Here's how the part is built. I have some questions about the finished solid (model axes, mm). Coordinates: 2 decimals unless noted, no trailing zeros. Write each loop counter-clockwise with the first axis right and the second up, starting at its lowest first coordinate (ties: lowest second). Pieces come first, ordered by that corner, then holes.
```python
from build123d import *

# Parameters (mm, degrees)
BOSS_EXTRUDE1_DEPTH      = 195
BOSS_EXTRUDE1_DEPTH_BACK = 195
BOSS_EXTRUDE1_START      = -20000
SKETCH1_W                = 640
SKETCH1_H                = 390
SKETCH2_W                = 300
SKETCH2_H                = 350
CUT_EXTRUDE1_DEPTH       = 20207.079530676
SKETCH3_W                = 290
SKETCH3_H                = 20
SKETCH3_W_2              = 600
SKETCH3_H_2              = 190
CUT_EXTRUDE2_DEPTH       = 20202.300081925
FILLET1_R                = 50
FILLET2_R                = 10
FILLET4_R                = 100


# Some blends are built 0.0001 mm under size
with BuildPart() as part:
    # Sketch1 → Boss-Extrude1 (new, two sides: drawn at the far end of the back side and taken through both)
    with BuildSketch(Plane.XY.offset(BOSS_EXTRUDE1_START - BOSS_EXTRUDE1_DEPTH_BACK)):
        Rectangle(SKETCH1_W, SKETCH1_H)
    extrude(amount=BOSS_EXTRUDE1_DEPTH + BOSS_EXTRUDE1_DEPTH_BACK)

    # Sketch2 → Cut-Extrude1 (cut, through all)
    with BuildSketch(Plane(origin=(320, 0, 0), x_dir=(0, 0, -1), z_dir=(1, 0, 0))):
        with Locations((20095, 0)):
            Rectangle(SKETCH2_W, SKETCH2_H)
    extrude(amount=-CUT_EXTRUDE1_DEPTH, mode=Mode.SUBTRACT)

    # Sketch3 → Cut-Extrude2 (cut, through all)
    with BuildSketch(Plane.XZ.offset(195)):
        with Locations((-155, -20165)):
            Rectangle(SKETCH3_W, SKETCH3_H)
        with Locations((155, -20165)):
            Rectangle(SKETCH3_W, SKETCH3_H)
        with Locations((0, -20040)):
            Rectangle(SKETCH3_W_2, SKETCH3_H_2)
    extrude(amount=-CUT_EXTRUDE2_DEPTH, mode=Mode.SUBTRACT)

    # Fillet1
    # the kernel refuses this fillet: 50 mm, written as the material it adds along each edge
    with BuildSketch(Plane(origin=(300, -195, -20135), x_dir=(-1, 0, 0), z_dir=(0, 1, 0)), Plane(origin=(-300, -195, -20135), x_dir=(0, 0, 1), z_dir=(0, 1, 0)), Plane(origin=(300, 175, -19945), x_dir=(0, 0, -1), z_dir=(0, 1, 0)), Plane(origin=(-300, -175, -19945), x_dir=(0, 1, 0), z_dir=(-1, 0, 0)), Plane(origin=(320, -175, -19945), x_dir=(0, 1, 0), z_dir=(-1, 0, 0)), Plane(origin=(-300, -195, -19945), x_dir=(1, 0, 0), z_dir=(0, 1, 0))) as fillet1_piece_1:
        with BuildLine():
            CenterArc((FILLET1_R, FILLET1_R), FILLET1_R, 180, 90)
            Line((0, FILLET1_R), (0, 0))
            Line((0, 0), (FILLET1_R, 0))
        make_face()
    extrude(amount=20)
    with BuildSketch(Plane(origin=(300, 175, -20135), x_dir=(0, 0, 1), z_dir=(0, 1, 0)), Plane(origin=(-300, 175, -20135), x_dir=(1, 0, 0), z_dir=(0, 1, 0)), Plane(origin=(300, -195, -19945), x_dir=(-1, 0, 0), z_dir=(0, 1, 0)), Plane(origin=(-300, 175, -19945), x_dir=(0, -1, 0), z_dir=(-1, 0, 0)), Plane(origin=(320, 175, -19945), x_dir=(0, -1, 0), z_dir=(-1, 0, 0)), Plane(origin=(-300, 175, -19945), x_dir=(0, 0, -1), z_dir=(0, 1, 0))) as fillet1_piece_2:
        with BuildLine():
            CenterArc((FILLET1_R, -FILLET1_R), FILLET1_R, 90, 90)
            Line((0, -FILLET1_R), (0, 0))
            Line((0, 0), (FILLET1_R, 0))
        make_face()
    extrude(amount=20)
    with BuildSketch(Plane(origin=(-300, -195, -20175), x_dir=(0, 0, 1), z_dir=(0, 1, 0))) as fillet1_piece_3:
        with BuildLine():
            CenterArc((50, 40), FILLET1_R, 180, 53.130102354)
            Line((0, 40), (0, 0))
            Line((0, 0), (20, 0))
        make_face()
    extrude(amount=20)
    with BuildSketch(Plane(origin=(-300, 175, -20175), x_dir=(1, 0, 0), z_dir=(0, 1, 0))) as fillet1_piece_4:
        with BuildLine():
            CenterArc((40, -50), FILLET1_R, 90, 53.130102354)
            Line((0, -20), (0, 0))
            Line((0, 0), (40, 0))
        make_face()
    extrude(amount=20)
    with BuildSketch(Plane(origin=(300, -195, -20175), x_dir=(-1, 0, 0), z_dir=(0, 1, 0))) as fillet1_piece_5:
        with BuildLine():
            CenterArc((40, 50), FILLET1_R, 216.869897646, 53.130102354)
            Line((0, 20), (0, 0))
            Line((0, 0), (40, 0))
        make_face()
    extrude(amount=20)
    with BuildSketch(Plane(origin=(300, 175, -20175), x_dir=(0, 0, 1), z_dir=(0, 1, 0))) as fillet1_piece_6:
        with BuildLine():
            CenterArc((50, -40), FILLET1_R, 126.869897646, 53.130102354)
            Line((0, -40), (0, 0))
            Line((0, 0), (20, 0))
        make_face()
    extrude(amount=20)
    with BuildSketch(Plane(origin=(320, -175, -19945), x_dir=(0, 1, 0), z_dir=(-1, 0, 0))) as fillet1_piece_7a_section:
        with BuildLine():
            CenterArc((FILLET1_R, FILLET1_R), FILLET1_R, 180, 90)
            Line((0, FILLET1_R), (0, 0))
            Line((0, 0), (FILLET1_R, 0))
        make_face()
    fillet1_piece_7a = extrude(amount=145, mode=Mode.PRIVATE)
    fillet1_piece_7a = split(fillet1_piece_7a, bisect_by=Plane(origin=(300, -175, -19945), z_dir=(-1, 0, 0)), keep=Keep.TOP, mode=Mode.PRIVATE)
    with BuildSketch(Plane(origin=(300, -195, -19945), x_dir=(-1, 0, 0), z_dir=(0, 1, 0))) as fillet1_piece_7b_section:
        with BuildLine():
            CenterArc((FILLET1_R, -FILLET1_R), FILLET1_R, 90, 90)
            Line((0, -FILLET1_R), (0, 0))
            Line((0, 0), (FILLET1_R, 0))
        make_face()
    fillet1_piece_7b = extrude(amount=145, mode=Mode.PRIVATE)
    fillet1_piece_7b = split(fillet1_piece_7b, bisect_by=Plane(origin=(300, -175, -19945), z_dir=(0, 1, 0)), keep=Keep.TOP, mode=Mode.PRIVATE)
    fillet1_piece_7 = fillet1_piece_7a & fillet1_piece_7b
    add(fillet1_piece_7)
    with BuildSketch(Plane(origin=(300, 50, -19945), x_dir=(0, 0, -1), z_dir=(0, 1, 0))) as fillet1_piece_8a_section:
        with BuildLine():
            CenterArc((FILLET1_R, FILLET1_R), FILLET1_R, 180, 90)
            Line((0, FILLET1_R), (0, 0))
            Line((0, 0), (FILLET1_R, 0))
        make_face()
    fillet1_piece_8a = extrude(amount=145, mode=Mode.PRIVATE)
    fillet1_piece_8a = split(fillet1_piece_8a, bisect_by=Plane(origin=(300, 175, -19945), z_dir=(0, -1, 0)), keep=Keep.TOP, mode=Mode.PRIVATE)
    with BuildSketch(Plane(origin=(320, 175, -19945), x_dir=(0, -1, 0), z_dir=(-1, 0, 0))) as fillet1_piece_8b_section:
        with BuildLine():
            CenterArc((FILLET1_R, -FILLET1_R), FILLET1_R, 90, 90)
            Line((0, -FILLET1_R), (0, 0))
            Line((0, 0), (FILLET1_R, 0))
        make_face()
    fillet1_piece_8b = extrude(amount=145, mode=Mode.PRIVATE)
    fillet1_piece_8b = split(fillet1_piece_8b, bisect_by=Plane(origin=(300, 175, -19945), z_dir=(-1, 0, 0)), keep=Keep.TOP, mode=Mode.PRIVATE)
    fillet1_piece_8 = fillet1_piece_8a & fillet1_piece_8b
    add(fillet1_piece_8)
    with BuildSketch(Plane(origin=(-300, 50, -19945), x_dir=(0, 0, -1), z_dir=(0, 1, 0))) as fillet1_piece_9a_section:
        with BuildLine():
            CenterArc((FILLET1_R, -FILLET1_R), FILLET1_R, 90, 90)
            Line((0, -FILLET1_R), (0, 0))
            Line((0, 0), (FILLET1_R, 0))
        make_face()
    fillet1_piece_9a = extrude(amount=145, mode=Mode.PRIVATE)
    fillet1_piece_9a = split(fillet1_piece_9a, bisect_by=Plane(origin=(-300, 175, -19945), z_dir=(0, -1, 0)), keep=Keep.TOP, mode=Mode.PRIVATE)
    with BuildSketch(Plane(origin=(-175, 175, -19945), x_dir=(0, -1, 0), z_dir=(-1, 0, 0))) as fillet1_piece_9b_section:
        with BuildLine():
            CenterArc((FILLET1_R, -FILLET1_R), FILLET1_R, 90, 90)
            Line((0, -FILLET1_R), (0, 0))
            Line((0, 0), (FILLET1_R, 0))
        make_face()
    fillet1_piece_9b = extrude(amount=145, mode=Mode.PRIVATE)
    fillet1_piece_9b = split(fillet1_piece_9b, bisect_by=Plane(origin=(-300, 175, -19945), z_dir=(1, 0, 0)), keep=Keep.TOP, mode=Mode.PRIVATE)
    fillet1_piece_9 = fillet1_piece_9a & fillet1_piece_9b
    add(fillet1_piece_9)
    with BuildSketch(Plane(origin=(-300, -195, -19945), x_dir=(1, 0, 0), z_dir=(0, 1, 0))) as fillet1_piece_10a_section:
        with BuildLine():
            CenterArc((FILLET1_R, FILLET1_R), FILLET1_R, 180, 90)
            Line((0, FILLET1_R), (0, 0))
            Line((0, 0), (FILLET1_R, 0))
        make_face()
    fillet1_piece_10a = extrude(amount=145, mode=Mode.PRIVATE)
    fillet1_piece_10a = split(fillet1_piece_10a, bisect_by=Plane(origin=(-300, -175, -19945), z_dir=(0, 1, 0)), keep=Keep.TOP, mode=Mode.PRIVATE)
    with BuildSketch(Plane(origin=(-175, -175, -19945), x_dir=(0, 1, 0), z_dir=(-1, 0, 0))) as fillet1_piece_10b_section:
        with BuildLine():
            CenterArc((FILLET1_R, FILLET1_R), FILLET1_R, 180, 90)
            Line((0, FILLET1_R), (0, 0))
            Line((0, 0), (FILLET1_R, 0))
        make_face()
    fillet1_piece_10b = extrude(amount=145, mode=Mode.PRIVATE)
    fillet1_piece_10b = split(fillet1_piece_10b, bisect_by=Plane(origin=(-300, -175, -19945), z_dir=(1, 0, 0)), keep=Keep.TOP, mode=Mode.PRIVATE)
    fillet1_piece_10 = fillet1_piece_10a & fillet1_piece_10b
    add(fillet1_piece_10)
    # the kernel refuses this fillet: 50 mm, written as the material it takes off along each edge
    with BuildSketch(Plane(origin=(320, -50, -20195), x_dir=(-1, 0, 0), z_dir=(0, -1, 0)), Plane(origin=(-320, -320, -20195), x_dir=(1, 0, 0), z_dir=(0, 1, 0)), Plane(origin=(320, 320, -20195), x_dir=(-1, 0, 0), z_dir=(0, -1, 0))) as fillet1_2_piece_1:
        with BuildLine():
            CenterArc((FILLET1_R, -FILLET1_R), FILLET1_R, 90, 90)
            Line((0, -FILLET1_R), (0, 0))
            Line((0, 0), (FILLET1_R, 0))
        make_face()
    extrude(amount=270, mode=Mode.SUBTRACT)
    with BuildSketch(Plane(origin=(-320, 50, -20195), x_dir=(0, 0, 1), z_dir=(0, 1, 0))) as fillet1_2_piece_2:
        with BuildLine():
            CenterArc((FILLET1_R, FILLET1_R), FILLET1_R, 180, 90)
            Line((0, FILLET1_R), (0, 0))
            Line((0, 0), (FILLET1_R, 0))
        make_face()
    extrude(amount=270, mode=Mode.SUBTRACT)

    # Fillet2
    fillet2_edges = [part.edges().sort_by_distance(p)[0] for p in [
        (-10, -185, -20175),
        (-10, 185, -20175),
        (10, -185, -20175),
        (10, 185, -20175),
        (10, 185, -20155),
        (10, -185, -20155),
        (-10, 185, -20155),
        (-10, -185, -20155),
    ]]
    fillet(fillet2_edges, radius=FILLET2_R - 0.0001)  # a hair under: the kernel refuses the full size

    # Fillet4
    fillet4_edges = [part.edges().sort_by_distance(p)[0] for p in [
        (-320, 0, -19805),
        (320, 0, -19805),
    ]]
    fillet(fillet4_edges, radius=FILLET4_R)


solid = part.part
```
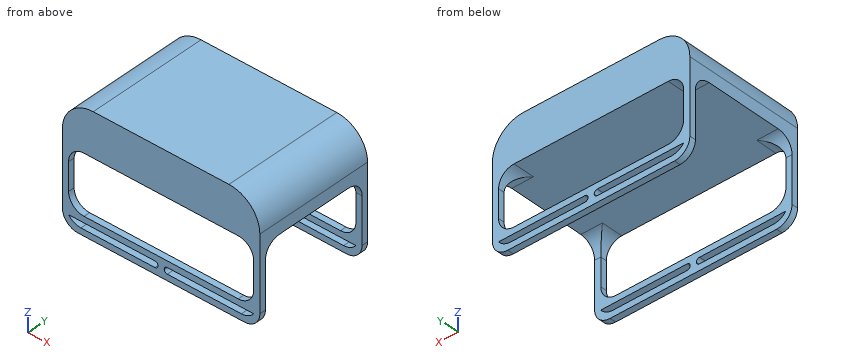
1) Imagine slicing it at D-D on y = 67.5. Please give me the cut outline in (x, z).
Values follow:
outline: (-320, -19945) - (320, -19945) - (320, -19905) arc R100 ccw to (220, -19805) - (-220, -19805) arc R100 ccw to (-320, -19905) - close
2) Will these pins go through, and if not, where does the flat tip stop? pin 1 (1.5 mm diameter, centred on x = 242, y = -119, fed in from +Z); pin 2 (4 mm diameter, centred on x = -234, y = 96.5, fed in from -Z).
Values follow:
pin 1: stops at z = -19807.28
pin 2: stops at z = -19945
3) Imagine slicing it at C-C on x = 1. Please give me the cut outline in (y, z), then the cut area to 3 significant figures.
Values follow:
outline: (-195, -20195) - (-175, -20195) - (-175, -20135) - (-195, -20135) - close; (-195, -19945) - (195, -19945) - (195, -19805) - (-195, -19805) - close; (175, -20195) - (195, -20195) - (195, -20135) - (175, -20135) - close
area: 57,000 mm2
4) I need wall thicknesses on probe 1 along Z at (x, y) = (131, -179); probe 2 along X at (y, z) = (-176, -20006.5); probe 3 along Z at (x, y) = (-63, -100). Which ranges of each line are inside material? Lowest first, please.
Values follow:
probe 1: z = -20195 to -20175, -20155 to -20135, -19945 to -19805
probe 2: x = -320 to -300, 300 to 320
probe 3: z = -19945 to -19805
5) Imagine slicing it at B-B on z = -20067. Please give me the cut outline in (x, y).
Values follow:
outline: (-320, -195) - (-300, -195) - (-300, -175) - (-320, -175) - close; (-320, 175) - (-300, 175) - (-300, 195) - (-320, 195) - close; (300, -195) - (320, -195) - (320, -175) - (300, -175) - close; (300, 175) - (320, 175) - (320, 195) - (300, 195) - close
6) Imagine slicing it at A-A on x = -136. Please give me the cut outline in (y, z), then the cut area to 3 significant figures.
Values follow:
outline: (-195, -20195) - (-175, -20195) - (-175, -20175) - (-195, -20175) - close; (-195, -20155) - (-175, -20155) - (-175, -20135) - (-195, -20135) - close; (-195, -19945) - (195, -19945) - (195, -19805) - (-195, -19805) - close; (175, -20195) - (195, -20195) - (195, -20175) - (175, -20175) - close; (175, -20155) - (195, -20155) - (195, -20135) - (175, -20135) - close
area: 56,200 mm2
